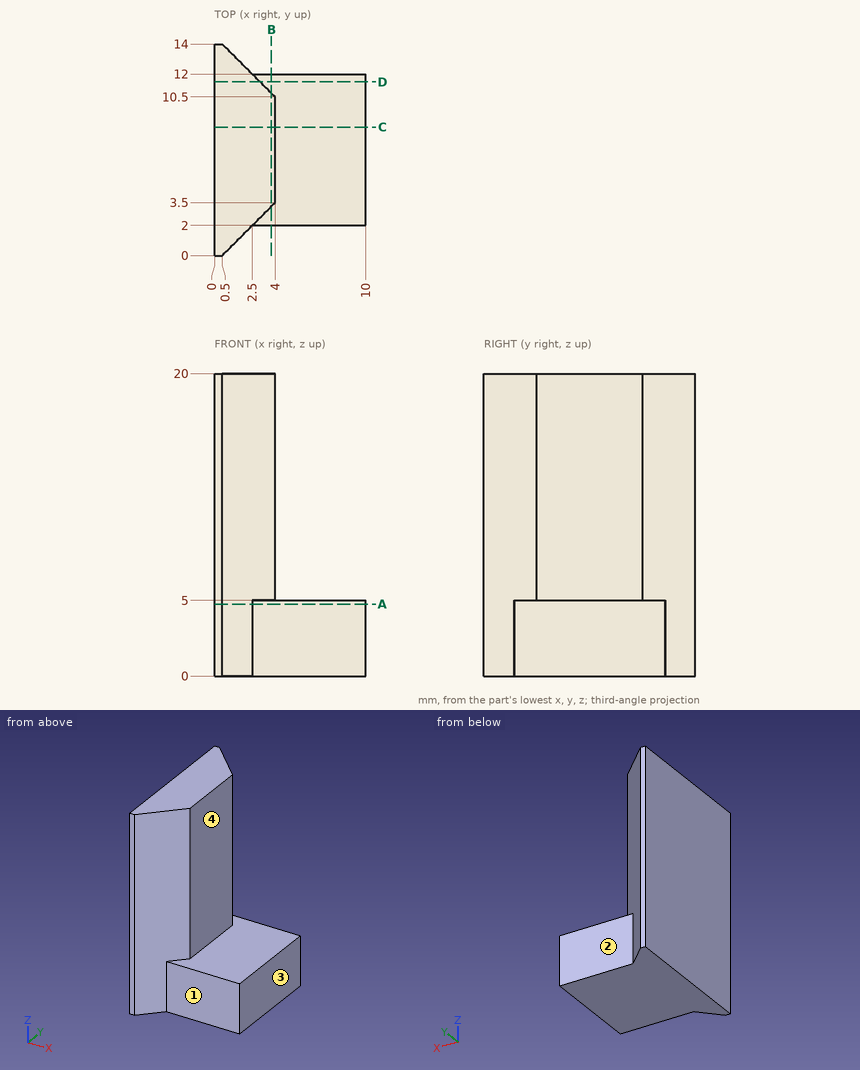
Could you check a few things on this drawing? It's one solid part, dimensions in mm from its lowest x, y, z. A direction names the side the tool comes from. Give positions to 0.01 mm unless a question says otherwise; leave off trailing zeros. Order: outer loops, then holes, each group sorted by start corner. A loop starts at its lowest first (then second) coordinate and runs counter-clockwise, first axis right, second up. Notation, with made-up numbers: (79, 19) - (108, 19) arc R31 ccw to (108, 49) - close; hole circle Ø7 at (-9, 56). An arc over 180 degrees is marked (long way). Return JSON: item names as keys, results as strings. Group by question number.
Q1. Please list where these lines run through material, in increasing order: line 1 along X through (y, z) = (8.25, 15); line 2 along Z through (x, y) = (5, 2.75); line 3 along X through (y, z) = (12.5, 18.5). Write a range as [from, to].
Q2. Which directions (+Z, -Z, +X, -X, +Y, -Y) give clear straight access to the entire face, cutting with the end or side of a thin tool? Please do the marked faces 1, 2, 3 and 4.
Q3. Suppose I cut it at B-B, the plane x = 3.75. Please give me the cut outline in (y, z), and give its area (4 significant figures).
Q4. Will these pins go through, and if not, where does the flat tip stop? pin 1 Ø2 at (x, y) = (4.5, 11.5) entering from +Z; pin 2 Ø1.5 at (x, z) = (5, 3.5) entering from +Y; pin 3 Ø2 at (y, z) = (7.5, 15.5) entering from +X.
Q5. Suppose I cut it at D-D, the plane y = 11.5. Please give me the cut outline in (x, z).
Q6. Suppose I cut it at C-C, the plane y = 8.5. Please give me the cut outline in (x, z), and give its area (3 significant figures).
Q7. Suppose I cut it at A-A, the plane z = 4.75. Please give me the cut outline in (x, y).
Resolved:
{
 "1": {"line 1": "x = [0, 4]", "line 2": "z = [0, 5]", "line 3": "x = [0, 2]"},
 "2": {"face 1": "+Z, -Z, +X, -Y", "face 2": "+Z, -Z, +X, +Y", "face 3": "+Z, -Z, +X, +Y, -Y", "face 4": "+Z, +X, +Y, -Y"},
 "3": {"outline": "(2, 0) - (12, 0) - (12, 5) - (10.75, 5) - (10.75, 20) - (3.25, 20) - (3.25, 5) - (2, 5) - close", "area": "162.5 mm2"},
 "4": {"pin 1": "stops at z = 5", "pin 2": "stops at y = 12", "pin 3": "stops at x = 4"},
 "5": {"outline": "(0, 0) - (10, 0) - (10, 5) - (3, 5) - (3, 20) - (0, 20) - close"},
 "6": {"outline": "(0, 0) - (10, 0) - (10, 5) - (4, 5) - (4, 20) - (0, 20) - close", "area": "110 mm2"},
 "7": {"outline": "(0, 0) - (0.5, 0) - (2.5, 2) - (10, 2) - (10, 12) - (2.5, 12) - (0.5, 14) - (0, 14) - close"}
}
